```python
from build123d import *

# Parameters (mm, degrees)
F1_DEPTH = 35
F2_R     = 5
F3_DEPTH = 2000
F5_DEPTH = 70
F6_W     = 30
F6_H     = 30
F7_DEPTH = 75


with BuildPart() as f1:
    # F0 (on Top) → F1 (new body)
    with BuildSketch(Plane.XY):
        with BuildLine():
            Line((-47.982599, 59.580382), (-62.982599, 59.580382))
            ThreePointArc((-62.982599, 59.580382), (-80.691861, -3.159854), (-59.585238, -64.840204))
            Line((-59.585238, -64.840204), (-44.585238, -64.840204))
            Line((-44.585238, -64.840204), (-44.585238, -49.840204))
            Line((-44.585238, -49.840204), (-47.585238, -49.840204))
            Line((-47.585238, -49.840204), (-50.585238, -49.840204))
            Line((-50.585238, -49.840204), (-50.585238, -50.840204))
            Line((-50.585238, -50.840204), (-47.585238, -50.840204))
            Line((-47.585238, -50.840204), (-47.585238, -59.677918))
            ThreePointArc((-47.585238, -59.677918), (-56.935757, -38.026074), (-62.037933, -14.999952))
            Line((-62.037933, -14.999952), (97.05541, -14.999952))
            Line((97.05541, -14.999952), (97.05541, 15.000048))
            Line((97.05541, 15.000048), (-62.114497, 15.000048))
            ThreePointArc((-62.114497, 15.000048), (-58.159644, 34.644429), (-51.106269, 53.40056))
            Line((-51.106269, 53.40056), (-50.99662, 45.580382))
            Line((-50.99662, 45.580382), (-53.982599, 45.580382))
            Line((-53.982599, 45.580382), (-53.982599, 44.580382))
            Line((-53.982599, 44.580382), (-47.982599, 44.580382))
            Line((-47.982599, 44.580382), (-47.982599, 59.580382))
        make_face()
    extrude(amount=F1_DEPTH)

    # F2 (on face) → F3 (cut)
    with BuildSketch(Plane.YZ.offset(97.05541)):
        with Locations((2.4e-05, 17.5)):
            Circle(F2_R)
    extrude(amount=-F3_DEPTH, mode=Mode.SUBTRACT)

    # F4 (on face) → F5 (cut)
    with BuildSketch(Plane.XZ.offset(14.999952)):
        Polygon((-17.94459, 20), (-17.94459, 17.5), (-17.94459, 15.032329), (97.05541, 15.032329), (97.05541, 20), align=None)
    extrude(amount=-F5_DEPTH, mode=Mode.SUBTRACT)

    # F6 (on face) → F7 (join)
    with BuildSketch(Plane(origin=(0, 0, 0), x_dir=(1, 0, 0), z_dir=(0, 0, -1))):
        with Locations((-29.112317, -4.8e-05)):
            Rectangle(F6_W, F6_H)
    extrude(amount=F7_DEPTH)


solid = f1.part
```
Here's how the part is built. I have some questions about the finished solid (model axes, mm). A direction names the side the tool comes from. Round coordinates to 2 decimals unless told otherwise and drop trailing zeros. Write each loop counter-clockwise with the first axis right and the second up, starting at its lowest first coordinate (ties: lowest second). Pieces come first, ordered by that corner, then holes.
Q1. If we mould it in two halves opening along X, with no side actions, what happens to faces 1 (the cylindrical face through (-58.24, 34.37, 17.26)), 2 (the cylindrical face through (-80.713, -2.233, 9.477)), 3 (the flat face through (39, 10, 15.032)), 4 (the flat face through (-44.585, -57, 17))? For each: +X half, -X half, draft (parallel to the pull), parting line (faces both ways), or undercut.
Q2. If we section it at A-A on x = 60.5: Write out the boundary of the cut face in (y, z), plus the area to 3 significant figures.
Q3. If we section it at B-B on z = 17.5: Write out the boundary of the cut face in (x, y), plus the area to 3 significant figures.
Q4. If we section it at C-C on z = 2.5: Write out the boundary of the cut face in (x, y), plus the area to 3 significant figures.
Q5. Please list where these lines run through material, in increasing order: probe 1 along Y at (x, z) = (-27.5, 17.5); probe 2 along Z at (x, y) = (30, 12.5); probe 3 along Z at (x, y) = (-68.5, 38).
Q6. Will these pins go through, and if not, where does the flat tip stop? P1, Ø11.5, axis at x = 26.5, y = 9, coming from the -Z side; P2, Ø2.5, axis at y = 8, z = 17.5, coming from the +X side; P3, Ø24, axis at y = -2, z = -47.5, coming from the -X side; P4, Ø1, axis at x = 68, z = 16.5, coming from the -Y side.
Q7. If we section it at D-D on x = -26.5: Write out the boundary of the cut face in (y, z).
Q8. Which directions (+Z, -Z, +X, -X, +Y, -Y) give clear straight access to the entire face, cutting with the end or side of a thin tool? Please do faces 5 (the flat face through (-17.945, 10, 18)), 6 (the flat face through (-44.112, 0, -37)), 7 (the flat face through (-47.983, 52, 17)), 8 (the flat face through (-14.112, 0, -37)).
Answer below:
1. face 1: undercut
1. face 2: -X half
1. face 3: draft
1. face 4: +X half
2. outline: (-15, 0) - (15, 0) - (15, 15.03) - (4.35, 15.03) arc R5 cw to (-4.35, 15.03) - (-15, 15.03) - close; (-15, 20) - (-4.33, 20) arc R5 cw to (4.33, 20) - (15, 20) - (15, 35) - (-15, 35) - close
2. area: 870 mm2
3. outline: (-80.63, -5) arc R109.45 ccw to (-59.59, -64.84) - (-44.59, -64.84) - (-44.59, -49.84) - (-50.59, -49.84) - (-50.59, -50.84) - (-47.59, -50.84) - (-47.59, -59.68) arc R124.57 cw to (-62.04, -15) - (-17.94, -15) - (-17.94, -5) - close; (-80.61, 5) - (-17.94, 5) - (-17.94, 15) - (-62.11, 15) arc R124.57 cw to (-51.11, 53.4) - (-51, 45.58) - (-53.98, 45.58) - (-53.98, 44.58) - (-47.98, 44.58) - (-47.98, 59.58) - (-62.98, 59.58) arc R109.45 ccw to start
3. area: 2,900 mm2
4. outline: (-62.98, 59.58) arc R109.45 ccw to (-59.59, -64.84) - (-44.59, -64.84) - (-44.59, -49.84) - (-50.59, -49.84) - (-50.59, -50.84) - (-47.59, -50.84) - (-47.59, -59.68) arc R124.57 cw to (-62.04, -15) - (97.06, -15) - (97.06, 15) - (-62.11, 15) arc R124.57 cw to (-51.11, 53.4) - (-51, 45.58) - (-53.98, 45.58) - (-53.98, 44.58) - (-47.98, 44.58) - (-47.98, 59.58) - close
4. area: 6,980 mm2
5. probe 1: y = -15 to -5, 5 to 15
5. probe 2: z = 0 to 15.03, 20 to 35
5. probe 3: z = 0 to 35
6. P1: stops at z = 0
6. P2: stops at x = -17.94
6. P3: stops at x = -44.11
6. P4: passes through
7. outline: (-15, -75) - (15, -75) - (15, 35) - (-15, 35) - close; hole circle Ø10 at (0, 17.5)
8. face 5: +X, +Y, -Y
8. face 6: -Z, -X, +Y, -Y
8. face 7: +Z, -Z, +X, +Y
8. face 8: -Z, +X, +Y, -Y
